Work out the finished part from the listing and answer in its coordinate system (mm). A direction names the side the tool comes from. Coordinates: 2 decimals unless noted, no trailing zeros. Loops run counter-clockwise (first coordinate to the right, second up) from the corner with the lowest first, then second, coordinate; pieces in that order, holes last. Notation, with made-up numbers: (50.25, 38) -> (76.25, 38) arc R23 ccw to (76.25, 74) -> close; hole circle Ø6 at (70.5, 1). An arc over 180 degrees is marked (long way). Use a Markdown table: item, result.
from build123d import *

# Parameters (mm, degrees)
SKETCH1_W           = 100
SKETCH1_H           = 100
BOSS_EXTRUDE1_DEPTH = 5
SKETCH2_R           = 20
BOSS_EXTRUDE2_DEPTH = 80
SHELL1_T            = -3


with BuildPart() as part:
    # Sketch1 → Boss-Extrude1 (new body)
    with BuildSketch(Plane(origin=(0, 0, 0), x_dir=(0, 0, -1), z_dir=(1, 0, 0))):
        Rectangle(SKETCH1_W, SKETCH1_H)
    extrude(amount=BOSS_EXTRUDE1_DEPTH)

    # Sketch2 → Boss-Extrude2 (add)
    with BuildSketch(Plane(origin=(5, 0, 0), x_dir=(0, 0, -1), z_dir=(1, 0, 0))):
        Circle(SKETCH2_R)
    extrude(amount=BOSS_EXTRUDE2_DEPTH)

    # Shell1
    shell1_openings = [part.faces().sort_by_distance(p)[0] for p in [
        (85, 0, 0),
    ]]
    offset(amount=SHELL1_T, openings=shell1_openings, kind=Kind.INTERSECTION)


solid = part.part
Q1. Determine the mould class of faces 1 (the cylindrical face through (44.44, -19.524, 4.336)), 2 (the flat face through (3, 0, 0)), 3 (the flat face through (2, -50, 1)) for opening direction Z: pulls with the +Z half, pulls with the -Z half, needs draft (parallel to the pull), parting line crosses it, or undercut.
Solved:
| item | result |
|---|---|
| face 1 | parting line crosses it |
| face 2 | undercut |
| face 3 | needs draft |
Q2. Section D-D on z = -26 is taken. Determine the outline of the cut face in (x, y), and give its area (3 significant figures).
Solved:
| item | result |
|---|---|
| outline | (0, -50) -> (5, -50) -> (5, 50) -> (0, 50) -> close |
| area | 500 mm² |
Q3. Section C-C on x = 10 is taken. Determine the outline of the cut face in (y, z).
Solved:
| item | result |
|---|---|
| outline | circle Ø40 at (0, 0); hole circle Ø34 at (0, 0) |
Q4. For faces 4 (the flat face through (2, 50, 1)), 5 (the cylindrical face through (43.426, 14.334, -9.139)), determine the directions among +Z, -Z, +X, -X, +Y, -Y from which every point of the face is accessible in a straight line to the end or side of a thin tool.
Solved:
| item | result |
|---|---|
| face 4 | +Z, -Z, +X, -X, +Y |
| face 5 | +X |
Q5. Section A-A on y = 0 is taken. Determine the outline of the cut face in (x, z), and give its area (3 significant figures).
Solved:
| item | result |
|---|---|
| outline | (0, -50) -> (5, -50) -> (5, -20) -> (85, -20) -> (85, -17) -> (3, -17) -> (3, 17) -> (85, 17) -> (85, 20) -> (5, 20) -> (5, 50) -> (0, 50) -> close |
| area | 912 mm² |
Q6. Consider line 1 (Y direction, x = 51, z = 0); line 2 (X direction, y = 17.5, z = -40); line 3 (X direction, y = -13, z = 7.5). Determine where each line is inside the solid, lowest interval first. Write a range as [from, to].
Solved:
| item | result |
|---|---|
| line 1 | [-20, -17], [17, 20] |
| line 2 | [0, 5] |
| line 3 | [0, 3] |
Q7. Given pin 1 Ø4 at (y, z) = (38, -15.5) entering from +X; pin 2 Ø1.5 at (x, z) = (31.5, -12) entering from -Y; pin 3 Ø10 at (y, z) = (-8, -2) entering from +X, each flat-ended and moving along its own axis, determine where each tip first touches the part or whether it passes through.
Solved:
| item | result |
|---|---|
| pin 1 | x = 5 |
| pin 2 | y = -16.54 |
| pin 3 | x = 3 |
